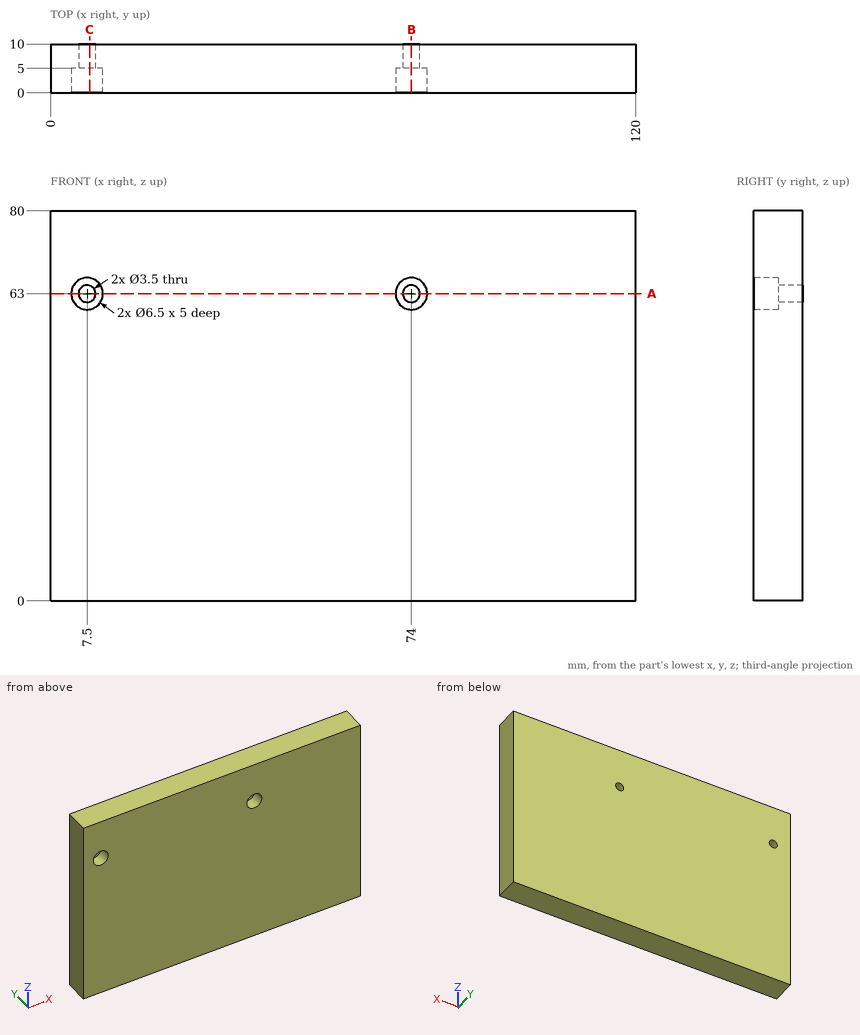
Input: dimensioned drawing with shaded views. Units: mm. Origin: part minimum x, y, z. Coordinates: 2 decimals unless noted, no trailing zeros. Write each loop counter-clockwise with the first axis right and the second up, starting at its lowest first coordinate (ties: lowest second). Pieces come first, ordered by that corner, then holes. Notation, with made-up numbers: (65, 85) -> (92, 85) arc R16 ccw to (92, 110) -> close; hole circle Ø1 at (2, -18.5). An arc over 180 degrees is marked (long way). Return JSON: item names as keys, results as strings. Group by question number.
1) Section query B-B, the plane x = 74. Return loops of the section in (y, z).
2) Ray query, line 1 along Z through (x, y) = (74, 8.45); line 2 along Z through (x, y) = (7.5, 3.55). Return the intervals inside material, ascending.
3) Section query C-C, the plane x = 8. Return loops of the section in (y, z).
4) Contact query for flat-ended pins moving along their axis: P1, Ø4, axis at x = 94.5, z = 60.5, coming from the -Y side; P2, Ø3, axis at x = 7, z = 64, coming from the -Y side. Output: stop coordinate, or through.
5) Section query A-A, the plane z = 63. Return loops of the section in (x, y).
From the geometry:
{
 "1": {"outline": "(0, 0) -> (10, 0) -> (10, 61.25) -> (5, 61.25) -> (5, 59.75) -> (0, 59.75) -> close; (0, 66.25) -> (5, 66.25) -> (5, 64.75) -> (10, 64.75) -> (10, 80) -> (0, 80) -> close"},
 "2": {"line 1": "0 to 61.25, 64.75 to 80", "line 2": "0 to 59.75, 66.25 to 80"},
 "3": {"outline": "(0, 0) -> (10, 0) -> (10, 61.32) -> (5, 61.32) -> (5, 59.79) -> (0, 59.79) -> close; (0, 66.21) -> (5, 66.21) -> (5, 64.68) -> (10, 64.68) -> (10, 80) -> (0, 80) -> close"},
 "4": {"P1": "y = 0", "P2": "y = 5"},
 "5": {"outline": "(0, 0) -> (4.25, 0) -> (4.25, 5) -> (5.75, 5) -> (5.75, 10) -> (0, 10) -> close; (9.25, 5) -> (10.75, 5) -> (10.75, 0) -> (70.75, 0) -> (70.75, 5) -> (72.25, 5) -> (72.25, 10) -> (9.25, 10) -> close; (75.75, 5) -> (77.25, 5) -> (77.25, 0) -> (120, 0) -> (120, 10) -> (75.75, 10) -> close"}
}
